```python
from build123d import *

# Parameters (mm, degrees)
SKETCH_1_R          = 3
EXTRUDE_1_DEPTH     = 3
SKETCH_2_W          = 10
SKETCH_2_H          = 10
SKETCH_2_R          = 0.8
EXTRUDE_2_DEPTH     = 1.5
SKETCH_5_W          = 10
SKETCH_5_H          = 2.5
CUT_EXTRUDE_1_DEPTH = 2.5
CUT_EXTRUDE_2_REACH = 15.748
FILLET_1_R          = 0.5
FILLET_2_R          = 0.2
CHAMFER_1_SIZE      = 0.2
SKETCH_3_R          = 3.977941141
EXTRUDE_3_DEPTH     = 0.4


with BuildPart() as part:
    # 草图1 → 凸台-拉伸1 (new body)
    with BuildSketch(Plane(origin=(0, 0, 0), x_dir=(0, 0, -1), z_dir=(1, 0, 0))):
        with BuildLine():
            Line((-5, 0), (-5, -8))
            Line((-5, -8), (5, -8))
            Line((5, -8), (5, 0))
            ThreePointArc((5, 0), (0, 5), (-5, 0))
        make_face()
        Circle(SKETCH_1_R, mode=Mode.SUBTRACT)
    extrude(amount=EXTRUDE_1_DEPTH)

    # 草图2 → 凸台-拉伸2 (add)
    with BuildSketch(Plane.XZ.offset(8)):
        with Locations((1.5, 0)):
            Rectangle(SKETCH_2_W, SKETCH_2_H)
        with Locations(Location((5, -1, 0), (0, 0, 270))):
            Circle(SKETCH_2_R, mode=Mode.SUBTRACT)
        with Locations(Location((-2, -1, 0), (0, 0, 270))):
            Circle(SKETCH_2_R, mode=Mode.SUBTRACT)
    extrude(amount=-EXTRUDE_2_DEPTH)

    # 草图5 → 切除-拉伸1 (cut)
    with BuildSketch(Plane.XZ.offset(8)):
        with Locations((1.5, 3.75)):
            Rectangle(SKETCH_5_W, SKETCH_5_H)
    extrude(amount=-CUT_EXTRUDE_1_DEPTH, mode=Mode.SUBTRACT)

    # 草图6 → 切除-拉伸2 (cut, up to next)
    with BuildSketch(Plane.ZY.offset(3.5), mode=Mode.PRIVATE) as cut_extrude_2_sk1:
        with BuildLine():
            Line((2.897366596, -6), (3.27705392, -6))
            Line((3.27705392, -6), (3.27705392, -8.325127743))
            Line((3.27705392, -8.325127743), (1, -8.325127743))
            Line((1, -8.325127743), (1, -8))
            ThreePointArc((1, -8), (2.378404875, -7.407669683), (2.897366596, -6))
        make_face()
    cut_extrude_2_tool1 = extrude(cut_extrude_2_sk1.sketch, amount=-CUT_EXTRUDE_2_REACH, mode=Mode.PRIVATE) & part.part
    add(cut_extrude_2_tool1.solids().sort_by_distance((-3.5, -7.575754, 2.569334))[0], mode=Mode.SUBTRACT)

    # 圆角1
    fillet_1_edges = [part.edges().sort_by_distance(p)[0] for p in [
        (3, -6.5, -1.25),
        (0, -6.5, -1.25),
    ]]
    fillet(fillet_1_edges, radius=FILLET_1_R)

    # 圆角2
    fillet_2_edges = [part.edges().sort_by_distance(p)[0] for p in [
        (-2, -6.5, -5),
        (-3.5, -7.25, -5),
        (6.5, -6.5, -1.25),
        (6.5, -7.25, -5),
        (6.5, -8, -2),
        (3, 5, 0),
        (-3.5, -6.5, -1.25),
        (3, -5.5, 3.75),
        (-3.5, -6.883095189, 2.5),
        (1.5, -5.5, 5),
        (0, -2.75, 5),
        (-2, -6.5, 2.5),
        (1.5, -5.5, 2.5),
        (6.5, -6.883095189, 2.5),
        (0, -5.5, 3.75),
        (0, 5, 0),
        (3, -2.75, 5),
        (-3.5, -8, -2),
        (1.5, -8, -5),
        (1.5, -7.266190379, 2.5),
        (-3.5, -7.806716397, 1.834936608),
        (6.5, -7.806716397, 1.834936608),
        (0, -5.75, 2.5),
        (0, -3, -5),
        (3, -5.75, 2.5),
        (3, -3, -5),
        (5, -6.5, 2.5),
        (5, -6.5, -5),
        (-0.146446609, -6.353553391, -5),
        (-0.146446609, -6.353553391, 2.5),
        (3.146446609, -6.353553391, -5),
        (3.146446609, -6.353553391, 2.5),
    ]]
    fillet(fillet_2_edges, radius=FILLET_2_R)

    # 倒角1
    chamfer_1_edges = [part.edges().sort_by_distance(p)[0] for p in [
        (0, 0, 3),
        (3, 0, 3),
    ]]
    chamfer(chamfer_1_edges, length=CHAMFER_1_SIZE)

    # 草图3 → 凸台-拉伸3 (add)
    with BuildSketch(Plane(origin=(3, 0, 0), x_dir=(0, 0, -1), z_dir=(1, 0, 0))):
        Circle(SKETCH_3_R)
    extrude(amount=-EXTRUDE_3_DEPTH)


solid = part.part
```
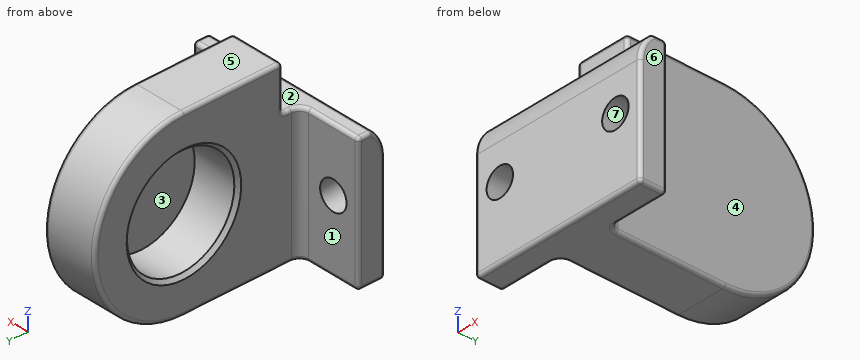
Verification items for the finished model (mm, model axes). Face numbers are marked on the shaded views. A direction names the side the tool comes from. Round coordinates to 2 decimals unless told otherwise and drop trailing zeros. Write each loop counter-clockwise with the first axis right and the second up, starting at its lowest first coordinate (ties: lowest second). Pieces come first, ordered by that corner, then holes. Notation, with made-up numbers: (3, 3.25) -> (38, 3.25) arc R19 cw to (38, 27.25) -> close; hole circle Ø5 at (-8, 69). An arc over 180 degrees is marked (long way). Write each question's results on one line, items separated by ' | '.
Q1. Thickness scan on probe 1 along X at (y, z) = (-7.4, -1); probe 2 along Z at (x, y) = (1.85, 0); probe 3 along X at (y, z) = (3.5, -0.25). Record the ranges inside material, lowest first.
Derived:
probe 1: x = -3.5 to -2.8, -1.2 to 4.2, 5.8 to 6.5 | probe 2: z = -5 to -3, 3 to 5 | probe 3: x = 0 to 3
Q2. Sectioned sample at A-A, the plane y = -7. Record the boundary of the cut face in (x, z).
Derived:
outline: (-3.5, -4.8) arc R0.2 ccw to (-3.3, -5) -> (6.3, -5) arc R0.2 ccw to (6.5, -4.8) -> (6.5, 2.3) arc R0.2 ccw to (6.3, 2.5) -> (-3.3, 2.5) arc R0.2 ccw to (-3.5, 2.3) -> close; hole circle Ø1.6 at (-2, -1); hole circle Ø1.6 at (5, -1)
Q3. Sectioned sample at D-D, the plane x = 6. Record the boundary of the cut face in (y, z), and give its area (3 significant figures).
Derived:
outline: (-8, -4.8) arc R0.2 ccw to (-7.8, -5) -> (-6.7, -5) arc R0.2 ccw to (-6.5, -4.8) -> (-6.5, 2.3) arc R0.2 ccw to (-6.7, 2.5) -> (-7.2, 2.5) arc R0.2 ccw to (-7.32, 2.45) arc R1.9 ccw to (-8, 1) -> close | area: 10.9 mm²
Q4. Sectioned sample at B-B, the plane x = -2. Record the boundary of the cut face in (y, z).
Derived:
outline: (-8, -4.8) arc R0.2 ccw to (-7.8, -5) -> (-6.7, -5) arc R0.2 ccw to (-6.5, -4.8) -> (-6.5, -1.8) -> (-8, -1.8) -> close; (-8, -0.2) -> (-6.5, -0.2) -> (-6.5, 2.3) arc R0.2 ccw to (-6.7, 2.5) -> (-7.2, 2.5) arc R0.2 ccw to (-7.32, 2.45) arc R1.9 ccw to (-8, 1) -> close
Q5. Go/stop test with flat-tipped pins: pin 1 Ø3 at (y, z) = (1.5, -1) entering from +X; pin 2 Ø1 at (x, z) = (4.5, 2.5) entering from +Y; pin 3 Ø0.7 at (x, y) = (0.5, -6) entering from +Z. Record where each tip stops, or that it passes through.
Derived:
pin 1: stops at x = 3 | pin 2: stops at y = -6.5 | pin 3: stops at z = 2.51
Q6. Draft check along X on the marked faces 5, 6 and 7. Enter one of: released by +X, released by -X, zero draft, split by the parting line, or undercut.
Derived:
face 5: zero draft | face 6: released by +X | face 7: undercut
Q7. Sectioned sample at C-C, the plane z = 0. Record the boundary of the cut face in (x, y).
Derived:
outline: (-3.5, -7.8) arc R0.2 ccw to (-3.3, -8) -> (6.3, -8) arc R0.2 ccw to (6.5, -7.8) -> (6.5, -6.7) arc R0.2 ccw to (6.3, -6.5) -> (3.5, -6.5) arc R0.5 cw to (3, -6) -> (3, 4.8) arc R0.2 ccw to (2.8, 5) -> (0.2, 5) arc R0.2 ccw to (0, 4.8) -> (0, 3.2) -> (0.2, 3) -> (2.6, 3) -> (2.6, -3) -> (0.2, -3) -> (0, -3.2) -> (0, -6) arc R0.5 cw to (-0.5, -6.5) -> (-3.3, -6.5) arc R0.2 ccw to (-3.5, -6.7) -> close
Q8. Access from +Z, -Z, +X, -X, +Y, -Y to the whole of each face (thin tool, end or side, straight path). Record for the marked faces 1, 2, 3 and 4.
Derived:
face 1: +Z, -Z, -X, +Y | face 2: +Z, +X, -X, -Y | face 3: -X | face 4: +Z, -Z, +X, +Y
